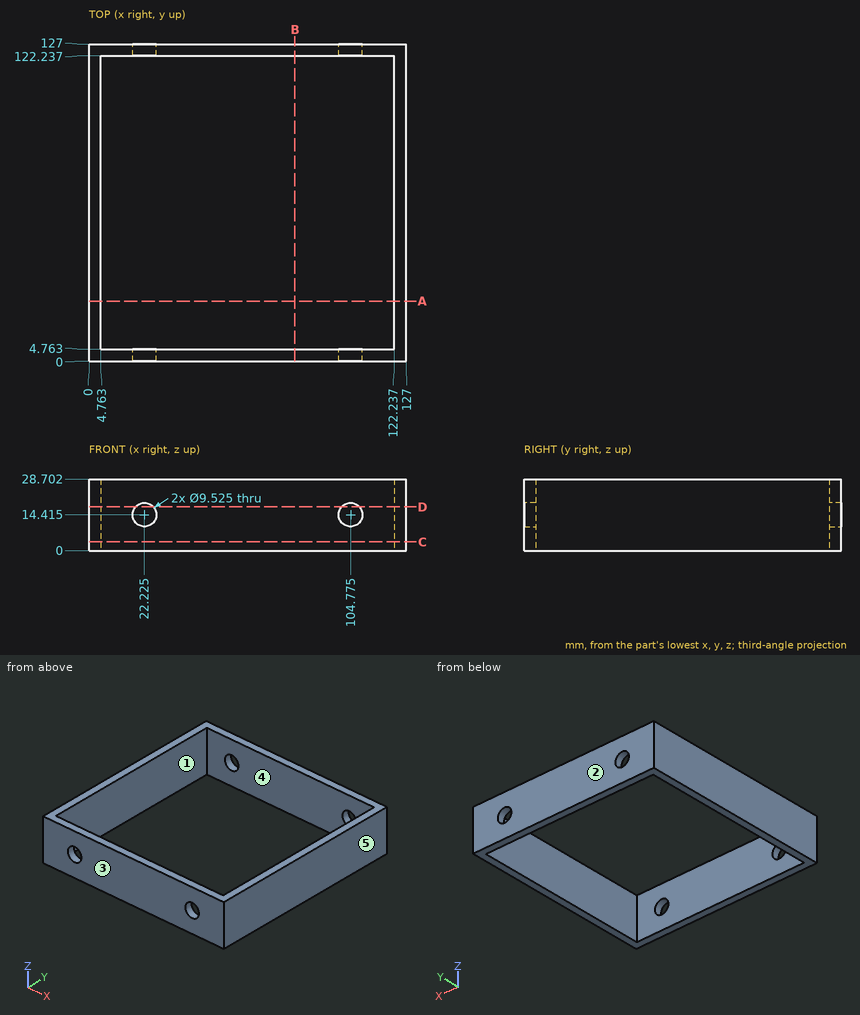
The drawing under review shows one solid part. Ordinate dimensions are in mm from its lowest x, y, z. A direction names the side the tool comes from. Round coordinates to 2 decimals unless told otherwise and drop trailing zeros. Write each loop counter-clockwise with the first axis right and the second up, starting at its lowest first coordinate (ties: lowest second). Pieces come first, ordered by that corner, then holes.
(1) We need section A-A on y = 24. Give the boundary of the cut face in (x, z).
(2) Mouldability with a two-part tool opening along X and no side actions: class the marked faces 3, 4 and 5 as +X half, -X half, draft (parallel to the pull), parting line (faces both ways), or undercut.
(3) We need section C-C on z = 3.5. Give the boundary of the cut face in (x, y), and give its area (3 significant figures).
(4) We need section D-D on z = 17.5. Give the boundary of the cut face in (x, y).
(5) Wall thickness on L1, parallel to Y at x = 46, z = 6.25: over which ranges is the line inside the solid? List them lowest first.
(6) Machinability: for the marked faces 1 and 2, which of the approach directions +Z, -Z, +X, -X, +Y, -Y give a long, thin tool a straight path to every point of the face, cutting with its end or side? Answer none if there is none.
Findings below:
1. outline: (0, 0) - (4.76, 0) - (4.76, 28.7) - (0, 28.7) - close; (122.24, 0) - (127, 0) - (127, 28.7) - (122.24, 28.7) - close
2. face 3: draft
2. face 4: undercut
2. face 5: +X half
3. outline: (0, 0) - (127, 0) - (127, 127) - (0, 127) - close; hole (4.76, 4.76) - (122.24, 4.76) - (122.24, 122.24) - (4.76, 122.24) - close
3. area: 2,330 mm2
4. outline: (0, 0) - (18.6, 0) - (18.6, 4.76) - (4.76, 4.76) - (4.76, 122.24) - (18.6, 122.24) - (18.6, 127) - (0, 127) - close; (25.85, 0) - (101.15, 0) - (101.15, 4.76) - (25.85, 4.76) - close; (25.85, 122.24) - (101.15, 122.24) - (101.15, 127) - (25.85, 127) - close; (108.4, 0) - (127, 0) - (127, 127) - (108.4, 127) - (108.4, 122.24) - (122.24, 122.24) - (122.24, 4.76) - (108.4, 4.76) - close
5. L1: y = 0 to 4.76, 122.24 to 127
6. face 1: +Z, -Z
6. face 2: +Z, -Z, +X, -X, +Y
